from build123d import *

# Parameters (mm, degrees)
CROQUIS1_R                   = 1.5
CROQUIS1_W                   = 2.95
CROQUIS1_H                   = 13.5
CROQUIS1_W_2                 = 13.5
CROQUIS1_H_2                 = 2.95
SALIENTE_EXTRUIR1_DEPTH      = 3
TALADRO_DE_MARGEN_PARA_M31_D = 3.4


with BuildPart() as part:
    # Croquis1 → Saliente-Extruir1 (new body)
    with BuildSketch(Plane(origin=(0, 0, 0), x_dir=(1, 0, 0), z_dir=(0, 1, 0))):
        with BuildLine():
            Line((-30, -38.4717102), (-30, 4.669623367))
            Line((-30, 4.669623367), (-32.892040435, 4.669623367))
            ThreePointArc((-32.892040435, 4.669623367), (-38.806634145, 10.584217077), (-32.892040435, 16.498810786))
            Line((-32.892040435, 16.498810786), (-30, 16.498810786))
            Line((-30, 16.498810786), (-30, 45))
            Line((-30, 45), (-30, 54))
            Line((-30, 54), (-32.892040435, 54))
            ThreePointArc((-32.892040435, 54), (-36.801169554, 55.882515512), (-37.766700191, 60.112516186))
            ThreePointArc((-37.766700191, 60.112516186), (-32.601856319, 63.859635989), (-27.068280751, 67.037065844))
            Line((-27.068280751, 67.037065844), (-15.492425724, 67.037065844))
            Line((-15.492425724, 67.037065844), (-15.492425724, 55.619045247))
            Line((-15.492425724, 55.619045247), (-15.492425724, 49.113101928))
            ThreePointArc((-15.492425724, 49.113101928), (-14.174406239, 45.931121412), (-10.992425724, 44.613101928))
            Line((-10.992425724, 44.613101928), (11.007574276, 44.613101928))
            ThreePointArc((11.007574276, 44.613101928), (14.189554792, 45.931121412), (15.507574276, 49.113101928))
            Line((15.507574276, 49.113101928), (15.507574276, 55.631560476))
            Line((15.507574276, 55.631560476), (15.507574276, 67.037065844))
            Line((15.507574276, 67.037065844), (27.068280751, 67.037065844))
            ThreePointArc((27.068280751, 67.037065844), (32.60050386, 63.860511342), (37.764196466, 60.114544216))
            ThreePointArc((37.764196466, 60.114544216), (36.799777556, 55.883328786), (32.89, 54))
            Line((32.89, 54), (30, 54))
            Line((30, 54), (30, 45))
            Line((30, 45), (30, 16.498810786))
            Line((30, 16.498810786), (32.75, 16.545073224))
            ThreePointArc((32.75, 16.545073224), (39.071015067, 10.224058157), (32.75, 3.90304309))
            Line((32.75, 3.90304309), (30, 3.90304309))
            Line((30, 3.90304309), (30, -38.4717102))
            ThreePointArc((30, -38.4717102), (0, -46.510185973), (-30, -38.4717102))
        make_face()
        with Locations(Location((-32.892040435, 10.584217077, 0), (0, 0, 270))):
            Circle(CROQUIS1_R, mode=Mode.SUBTRACT)
        with Locations(Location((32.75, 10.224058157, 0), (0, 0, 270))):
            Circle(CROQUIS1_R, mode=Mode.SUBTRACT)
        with Locations(Location((-32.892040435, 59, 0), (0, 0, 270))):
            Circle(CROQUIS1_R, mode=Mode.SUBTRACT)
        with Locations(Location((32.89, 59, 0), (0, 0, 270))):
            Circle(CROQUIS1_R, mode=Mode.SUBTRACT)
        with Locations((-26.775, -9.34695691)):
            Rectangle(CROQUIS1_W, CROQUIS1_H, mode=Mode.SUBTRACT)
        with Locations((26.775, -9.34695691)):
            Rectangle(CROQUIS1_W, CROQUIS1_H, mode=Mode.SUBTRACT)
        with Locations((5.25, -27.475)):
            Rectangle(CROQUIS1_W_2, CROQUIS1_H_2, mode=Mode.SUBTRACT)
    extrude(amount=SALIENTE_EXTRUIR1_DEPTH)

    # Taladro de margen para M31 (through all)
    with Locations(Plane(origin=(-27.009031687, 3, 36.020030417), x_dir=(0, 0, 1), z_dir=(0, 1, 0))):
        with Locations((0, 0), (6.887961272, 27.009031687), (0, 54.018063374)):
            Hole(TALADRO_DE_MARGEN_PARA_M31_D / 2)


solid = part.part
Input: part model. Units: mm. Frame: model coordinates. A direction names the side the tool comes from. Give positions to 0.01 mm unless a question says otherwise; leave off trailing zeros. Loops run counter-clockwise (first coordinate to the right, second up) from the corner with the lowest first, then second, coordinate; pieces in that order, holes last. Notation, with made-up numbers: (74.25, 10) -> (115.25, 10) arc R30 ccw to (115.25, 32) -> close; hole circle Ø2 at (-24.75, 47). An arc over 180 degrees is marked (long way). Answer as a JSON object with one key per item and string values. Group by question number.
Item 1: Pin query (flat end, axial travel): P1, Ø1.5, axis at y = 1.5, z = -55, coming from the +X side; P2, Ø0.9, axis at x = -31.5, y = 1, coming from the +Z side; P3, Ø1.5, axis at y = 1, z = -61.5, coming from the -X side. Return the tip coordinate at first contact, or that it passes through.
Item 2: Cut plane B-B, the plane z = -59. Return the cut outline in (x, y).
Item 3: Cut plane C-C, the plane z = 0. Return the cut outline in (x, y), and give its area (3 significant figures).
Item 4: Cut plane D-D, the plane y = 0.9. State how many separate pieces and enclosed holes the cut face has, and give its area (3 significant figures).
Item 5: Pull-direction query (X, two-part tool) for faces 5 (the cylindrical face through (0.44, 1.48, 46.51)), 6 (the cylindrical face through (14.154, 1.479, -45.896)), 7 (the flat face through (-30, 1, -35)); classes: released by +X, released by -X, zero draft, split by the parting line, or undercut.
Item 6: Line query: probe 1 along X at (y, z) = (1.5, 11.5); probe 2 along X at (y, z) = (0.85, -59); probe 3 along X at (y, z) = (2.8, -41.5). Output: solid intervals per line, ascending.
Item 7: Cut plane A-A, the plane x = 0. Return the cut outline in (y, z), and give its area (3 significant figures).
Item 8: Reachability of faces 1 (the flat face through (0, 1, -44.613)), 2 (the flat face through (31, 1, -54)), 3 (the flat face through (5, 1, 28.95)), 4 (the cylindrical face through (-38.805, 1.479, -10.454)) from +Z, -Z, +X, -X, +Y, -Y: full face, straight path, thin tool, end or side. Return the list, or none.
Checks:
{
 "1": {"P1": "stops at x = 36.69", "P2": "stops at z = -4.67", "P3": "stops at x = -36.97"},
 "2": {"outline": "(-37.89, 0) -> (-34.39, 0) -> (-34.39, 3) -> (-37.89, 3) -> close; (-31.39, 0) -> (-15.49, 0) -> (-15.49, 3) -> (-31.39, 3) -> close; (15.51, 0) -> (31.39, 0) -> (31.39, 3) -> (15.51, 3) -> close; (34.39, 0) -> (37.89, 0) -> (37.89, 3) -> (34.39, 3) -> close"},
 "3": {"outline": "(-30, 0) -> (30, 0) -> (30, 3) -> (-30, 3) -> close", "area": "180 mm²"},
 "4": {"separate pieces": "1", "enclosed holes": "10", "area": "6,110 mm²"},
 "5": {"face 5": "split by the parting line", "face 6": "undercut", "face 7": "released by -X"},
 "6": {"probe 1": "x = -30 to -28.25, -25.3 to 25.3, 28.25 to 30", "probe 2": "x = -37.89 to -34.39, -31.39 to -15.49, 15.51 to 31.39, 34.39 to 37.89", "probe 3": "x = -30 to 30"},
 "7": {"outline": "(0, -44.61) -> (3, -44.61) -> (3, 26) -> (0, 26) -> close; (0, 28.95) -> (3, 28.95) -> (3, 41.21) -> (0, 41.21) -> close; (0, 44.61) -> (3, 44.61) -> (3, 46.51) -> (0, 46.51) -> close", "area": "254 mm²"},
 "8": {"face 1": "-Z, +Y, -Y", "face 2": "+X, +Y, -Y", "face 3": "+Y, -Y", "face 4": "-X, +Y, -Y"}
}
